For this review, take the finished solid that the model builds, in its own axes (mm). A direction names the side the tool comes from. Give positions to 0.01 mm unless a question says otherwise; leave off trailing zeros. Loops run counter-clockwise (first coordinate to the right, second up) from the corner with the lowest first, then second, coordinate; pieces in that order, holes last. Notation, with made-up numbers: (18.25, 17) - (75.25, 17) arc R13 cw to (75.25, 31) - close; hole circle Ø2 at (21.25, 11). An arc over 180 degrees is marked (long way). Put each result on its own line as item: value.
from build123d import *

# Parameters (mm, degrees)
SKETCH2_R           = 2
BOSS_EXTRUDE1_DEPTH = 1.5
BOSS_EXTRUDE2_DEPTH = 16
BOSS_EXTRUDE3_START = -1
BOSS_EXTRUDE3_DEPTH = 1
CHAMFER1_SIZE       = 1.5


with BuildPart() as part:
    # Sketch2 → Boss-Extrude1 (new, symmetric)
    with BuildSketch(Plane.XY):
        with BuildLine():
            Line((-15.307106781, 11.707106781), (-23.954546191, 3.059667371))
            ThreePointArc((-23.954546191, 3.059667371), (-25, 0), (-23.954546191, -3.059667371))
            Line((-23.954546191, -3.059667371), (-15.307106781, -11.707106781))
            ThreePointArc((-15.307106781, -11.707106781), (-14.982683432, -11.923879533), (-14.6, -12))
            Line((-14.6, -12), (14.6, -12))
            ThreePointArc((14.6, -12), (14.982683432, -11.923879533), (15.307106781, -11.707106781))
            Line((15.307106781, -11.707106781), (23.954546191, -3.059667371))
            ThreePointArc((23.954546191, -3.059667371), (25, 0), (23.954546191, 3.059667371))
            Line((23.954546191, 3.059667371), (15.307106781, 11.707106781))
            ThreePointArc((15.307106781, 11.707106781), (14.982683432, 11.923879533), (14.6, 12))
            Line((14.6, 12), (-14.6, 12))
            ThreePointArc((-14.6, 12), (-14.982683432, 11.923879533), (-15.307106781, 11.707106781))
        make_face()
        with Locations((-20, 0)):
            Circle(SKETCH2_R, mode=Mode.SUBTRACT)
        with Locations(Location((20, 0, 0), (0, 0, 180))):
            Circle(SKETCH2_R, mode=Mode.SUBTRACT)
        with BuildLine():
            Line((-11.271320344, -3.878679656), (-7.878679656, -7.271320344))
            ThreePointArc((-7.878679656, -7.271320344), (-6.90540961, -7.921638598), (-5.757359313, -8.15))
            Line((-5.757359313, -8.15), (5.757359313, -8.15))
            ThreePointArc((5.757359313, -8.15), (6.90540961, -7.921638598), (7.878679656, -7.271320344))
            Line((7.878679656, -7.271320344), (11.271320344, -3.878679656))
            ThreePointArc((11.271320344, -3.878679656), (11.921638598, -2.90540961), (12.15, -1.757359313))
            Line((12.15, -1.757359313), (12.15, 5.15))
            ThreePointArc((12.15, 5.15), (11.271320344, 7.271320344), (9.15, 8.15))
            Line((9.15, 8.15), (-9.15, 8.15))
            ThreePointArc((-9.15, 8.15), (-11.271320344, 7.271320344), (-12.15, 5.15))
            Line((-12.15, 5.15), (-12.15, -1.757359313))
            ThreePointArc((-12.15, -1.757359313), (-11.921638598, -2.90540961), (-11.271320344, -3.878679656))
        make_face(mode=Mode.SUBTRACT)
    extrude(amount=BOSS_EXTRUDE1_DEPTH, both=True)

    # Sketch3 → Boss-Extrude2 (add)
    with BuildSketch(Plane(origin=(0, 0, -1.5), x_dir=(-1, 0, 0), z_dir=(0, 0, -1))):
        with BuildLine():
            Line((-9.15, 9.25), (9.15, 9.25))
            ThreePointArc((9.15, 9.25), (12.049137803, 8.049137803), (13.25, 5.15))
            Line((13.25, 5.15), (13.25, -1.757359313))
            ThreePointArc((13.25, -1.757359313), (12.937906083, -3.326361386), (12.049137803, -4.656497116))
            Line((12.049137803, -4.656497116), (8.656497116, -8.049137803))
            ThreePointArc((8.656497116, -8.049137803), (7.326361386, -8.937906083), (5.757359313, -9.25))
            Line((5.757359313, -9.25), (-5.757359313, -9.25))
            ThreePointArc((-5.757359313, -9.25), (-7.326361386, -8.937906083), (-8.656497116, -8.049137803))
            Line((-8.656497116, -8.049137803), (-12.049137803, -4.656497116))
            ThreePointArc((-12.049137803, -4.656497116), (-12.937906083, -3.326361386), (-13.25, -1.757359313))
            Line((-13.25, -1.757359313), (-13.25, 5.15))
            ThreePointArc((-13.25, 5.15), (-12.049137803, 8.049137803), (-9.15, 9.25))
        make_face()
        with BuildLine():
            Line((12.15, 5.15), (12.15, -1.757359313))
            ThreePointArc((12.15, -1.757359313), (11.921638598, -2.90540961), (11.271320344, -3.878679656))
            Line((11.271320344, -3.878679656), (7.878679656, -7.271320344))
            ThreePointArc((7.878679656, -7.271320344), (6.90540961, -7.921638598), (5.757359313, -8.15))
            Line((5.757359313, -8.15), (-5.757359313, -8.15))
            ThreePointArc((-5.757359313, -8.15), (-6.90540961, -7.921638598), (-7.878679656, -7.271320344))
            Line((-7.878679656, -7.271320344), (-11.271320344, -3.878679656))
            ThreePointArc((-11.271320344, -3.878679656), (-11.921638598, -2.90540961), (-12.15, -1.757359313))
            Line((-12.15, -1.757359313), (-12.15, 5.15))
            ThreePointArc((-12.15, 5.15), (-11.271320344, 7.271320344), (-9.15, 8.15))
            Line((-9.15, 8.15), (9.15, 8.15))
            ThreePointArc((9.15, 8.15), (11.271320344, 7.271320344), (12.15, 5.15))
        make_face(mode=Mode.SUBTRACT)
    extrude(amount=BOSS_EXTRUDE2_DEPTH)

    # Sketch4 → Boss-Extrude3 (add)
    with BuildSketch(Plane(origin=(0, 0, -17.5), x_dir=(-1, 0, 0), z_dir=(0, 0, -1)).offset(BOSS_EXTRUDE3_START)):
        with BuildLine():
            Line((9.15, 9.25), (-9.15, 9.25))
            ThreePointArc((-9.15, 9.25), (-12.049137803, 8.049137803), (-13.25, 5.15))
            Line((-13.25, 5.15), (-13.25, -1.757359313))
            ThreePointArc((-13.25, -1.757359313), (-12.937906083, -3.326361386), (-12.049137803, -4.656497116))
            Line((-12.049137803, -4.656497116), (-8.656497116, -8.049137803))
            ThreePointArc((-8.656497116, -8.049137803), (-7.326361386, -8.937906083), (-5.757359313, -9.25))
            Line((-5.757359313, -9.25), (5.757359313, -9.25))
            ThreePointArc((5.757359313, -9.25), (7.326361386, -8.937906083), (8.656497116, -8.049137803))
            Line((8.656497116, -8.049137803), (12.049137803, -4.656497116))
            ThreePointArc((12.049137803, -4.656497116), (12.937906083, -3.326361386), (13.25, -1.757359313))
            Line((13.25, -1.757359313), (13.25, 5.15))
            ThreePointArc((13.25, 5.15), (12.049137803, 8.049137803), (9.15, 9.25))
        make_face()
    extrude(amount=BOSS_EXTRUDE3_DEPTH)

    # Chamfer1
    chamfer1_edges = [part.edges().sort_by_distance(p)[0] for p in [
        (22, 0, 1.5),
        (-22, 0, 1.5),
    ]]
    chamfer(chamfer1_edges, length=CHAMFER1_SIZE)


solid = part.part
1) Take a section at B-B on z = -11.75. State the section outline as (x, y) points.
Geometry check:
outline: (-13.25, -1.76) arc R4.1 ccw to (-12.05, -4.66) - (-8.66, -8.05) arc R4.1 ccw to (-5.76, -9.25) - (5.76, -9.25) arc R4.1 ccw to (8.66, -8.05) - (12.05, -4.66) arc R4.1 ccw to (13.25, -1.76) - (13.25, 5.15) arc R4.1 ccw to (9.15, 9.25) - (-9.15, 9.25) arc R4.1 ccw to (-13.25, 5.15) - close; hole (-12.15, -1.76) arc R3 ccw to (-11.27, -3.88) - (-7.88, -7.27) arc R3 ccw to (-5.76, -8.15) - (5.76, -8.15) arc R3 ccw to (7.88, -7.27) - (11.27, -3.88) arc R3 ccw to (12.15, -1.76) - (12.15, 5.15) arc R3 ccw to (9.15, 8.15) - (-9.15, 8.15) arc R3 ccw to (-12.15, 5.15) - close
2) Draft analysis for pull direction X (two halves, no side actions). For faces 1 (the face through (11.915, -2.921, -7.374)), 2 (the face through (0, -12, 0)), 3 (the face through (-12, 8.1, -9.4)), 4 (the face through (11.29, 7.25, -7.37)), state which applies: pulls with the +X half, pulls with the -X half, needs draft (parallel to the pull), parting line crosses it, or undercut.
Geometry check:
face 1: undercut
face 2: needs draft
face 3: pulls with the -X half
face 4: undercut
3) Take a section at C-C on x = 4. State the section outline as (y, z) points, and give its area (3 significant figures).
Geometry check:
outline: (-12, -1.5) - (-9.25, -1.5) - (-9.25, -17.5) - (9.25, -17.5) - (9.25, -1.5) - (12, -1.5) - (12, 1.5) - (8.15, 1.5) - (8.15, -16.5) - (-8.15, -16.5) - (-8.15, 1.5) - (-12, 1.5) - close
area: 74.6 mm²
4) For faces 5 (the face through (12.1, 8, -9.4)), 6 (the face through (0, -8.15, -7)), 7 (the face through (13.25, 2, -9)), 8 (the face through (7.306, -8.946, -9.388)), 9 (the face through (-12.946, -3.306, -9.388)), list the 3-axis set-ups (+Z, -Z, +X, -X, +Y, -Y) from which the entire face can be reached by the end or side of a thin tool; tool diameter is ignored.
Geometry check:
face 5: -Z, +X, +Y
face 6: +Z
face 7: -Z, +X, +Y, -Y
face 8: -Z, +X, -Y
face 9: -Z, -X, -Y
5) Insertion check: pin 1 Ø2 at (y, z) = (2, -5.5) entering from +X; pin 2 Ø5 at (x, z) = (0.5, -7.5) entering from +Y; pin 3 Ø5 at (x, y) = (20, 0) entering from +Z. Each pin has a flat end and moves straight along its axis. Give the tip position at first contact, or say it passes through.
Geometry check:
pin 1: stops at x = 13.25
pin 2: stops at y = 9.25
pin 3: stops at z = 0.5
6) Take a section at A-A on y = 0. State the section outline as (x, z) points, and give its area (3 significant figures).
Geometry check:
outline: (-25, -1.5) - (-22, -1.5) - (-22, 0) - (-23.5, 1.5) - (-25, 1.5) - close; (-18, -1.5) - (-13.25, -1.5) - (-13.25, -17.5) - (13.25, -17.5) - (13.25, -1.5) - (18, -1.5) - (18, 0) - (16.5, 1.5) - (12.15, 1.5) - (12.15, -16.5) - (-12.15, -16.5) - (-12.15, 1.5) - (-16.5, 1.5) - (-18, 0) - close; (22, -1.5) - (25, -1.5) - (25, 1.5) - (23.5, 1.5) - (22, 0) - close
area: 108 mm²
7) Take a section at D-D on x = 20. State the section outline as (y, z) points, and give its area (3 significant figures).
Geometry check:
outline: (-7.01, -1.5) - (-2, -1.5) - (-2, 0) - (-3.5, 1.5) - (-7.01, 1.5) - close; (2, -1.5) - (7.01, -1.5) - (7.01, 1.5) - (3.5, 1.5) - (2, 0) - close
area: 27.8 mm²
8) Wall thickness on line 1 (X direction, y = -0.5, z = -13.75); line 2 (X direction, y = 1.75, z = 0.5); line 3 (Z direction, x = 12.5, y = 11.25): over which ranges is each line inside the solid? List them lowest first.
Geometry check:
line 1: x = -13.25 to -12.15, 12.15 to 13.25
line 2: x = -24.68 to -21.79, -18.21 to -12.15, 12.15 to 18.21, 21.79 to 24.68
line 3: z = -1.5 to 1.5
